```python
from build123d import *

# Parameters (mm, degrees)
F1_DEPTH = 25
F2_R     = 4
F3_DEPTH = 132.5
F4_R     = 4
F4_R_2   = 3.9797420395
F5_DEPTH = 8


with BuildPart() as f1:
    # F0 (on Top) → F1 (new body)
    with BuildSketch(Plane.XY):
        Polygon((45, 0), (0, 0), (0, 170), (-5, 170), (-5, -5), (50, -5), (50, 170), (45, 170), align=None)
    extrude(amount=F1_DEPTH)

    # F2 (on face) → F3 (cut)
    with BuildSketch(Plane(origin=(-5, 0, 0), x_dir=(0, -1, 0), z_dir=(-1, 0, 0))):
        with Locations((-160, 12.5)):
            Circle(F2_R)
    extrude(amount=-F3_DEPTH, mode=Mode.SUBTRACT)

    # F4 (on face) → F5 (join)
    with BuildSketch(Plane.YZ.offset(50)):
        Polygon((163.8578503757, 19.1819928586), (156.1421496243, 19.1819928586), (152.2842992487, 12.5), (156.1421496243, 5.8180071414), (163.8578503757, 5.8180071414), (167.7157007513, 12.5), align=None)
        with Locations((160, 12.5)):
            Circle(F4_R, mode=Mode.SUBTRACT)
        with Locations((160, 12.5)):
            Circle(F4_R)
        with Locations((160, 12.5)):
            Circle(F4_R_2, mode=Mode.SUBTRACT)
    extrude(amount=F5_DEPTH)


solid = f1.part
```
CAD build for the part. Positions are in the model's coordinates, mm. A direction names the side the tool comes from. Give positions to 0.01 mm unless a question says otherwise; leave off trailing zeros. Order: outer loops, then holes, each group sorted by start corner. A loop starts at its lowest first (then second) coordinate and runs counter-clockwise, first axis right, second up.
(1) Tool access for faces 1 (the flat face through (53.94, 154.24, 15.89)), 2 (the flat face through (54, 160, 5.818)), 3 (the flat face through (54, 160, 19.182)), 4 (the flat face through (53.944, 165.814, 15.794)), 5 (the flat face through (45, 86, 12)): list every direction of +Z, -Z, +X, -X, +Y, -Y with a clear straight run to the whole face (end or side of a thin tool).
(2) Mould opens along Z. For faces 6 (the cylindrical face through (47.465, 156.185, 13.701)), 7 (the flat face through (0, 84, 12)), 8 (the cylindrical face through (53.944, 156.024, 12.675)), 9 (the flat face through (53.94, 165.76, 9.11)) say: released by +Z, released by -Z, zero draft, split by the parting line, or undercut.
(3) Drill centre lines: L1, parallel to X at y = 24, z = 12.5; L2, parallel to Z at x = 54, y = 160; L3, parallel to Z at x = 49, y = 160. Where is each one in solid material? Low to high.
(4) Saw through at D-D, the plane x = 35. Give the cut face in (y, z).
(5) Saw through at C-C, the plane z = 3.25. Give the cut face in (x, y), then the cut area to 4 significant figures.
(6) Flat gauge pins, fed straight in: pin 1 (1 mm diameter, centred on y = 78, z = 15, fed in from +X); pin 2 (13 mm diameter, centred on y = 160, z = 12.5, fed in from +X); pin 3 (6 mm diameter, centred on x = 56, y = 158.5, fed in from -Z); pin 4 (8.5 mm diameter, centred on x = 55, y = 159.5, fed in from +Z). Where does each tip first touch, or does it go through?
(7) Saw through at B-B, the plane y = 66. Give the cut face in (x, z), then the cut area to 3 significant figures.
(8) Saw through at A-A, the plane y = 160. State how many separate pieces and enclosed holes the cut face has, then the cut area to 3 significant figures.
Results found:
1. face 1: +Z, +X, -Y
1. face 2: -Z, +X, +Y, -Y
1. face 3: +Z, +X, +Y, -Y
1. face 4: +Z, +X, +Y
1. face 5: +Z, -Z, +Y
2. face 6: undercut
2. face 7: zero draft
2. face 8: undercut
2. face 9: released by -Z
3. L1: x = -5 to 0, 45 to 50
3. L2: z = 5.82 to 8.52, 16.48 to 19.18
3. L3: z = 0 to 8.5, 16.5 to 25
4. outline: (-5, 0) - (0, 0) - (0, 25) - (-5, 25) - close
5. outline: (-5, -5) - (50, -5) - (50, 170) - (45, 170) - (45, 0) - (0, 0) - (0, 170) - (-5, 170) - close
5. area: 1,975 mm2
6. pin 1: stops at x = 50
6. pin 2: stops at x = 58
6. pin 3: stops at z = 5.82
6. pin 4: stops at z = 19.18
7. outline: (-5, 0) - (0, 0) - (0, 25) - (-5, 25) - close; (45, 0) - (50, 0) - (50, 25) - (45, 25) - close
7. area: 250 mm2
8. separate pieces: 4
8. enclosed holes: 0
8. area: 213 mm2
